Source: CAD feature listing. Evaluate the final solid. Frame: model axes, mm. A direction names the side the tool comes from. Coordinates: 2 decimals unless noted, no trailing zeros. Write each loop counter-clockwise with the first axis right and the second up, starting at its lowest first coordinate (ties: lowest second). Pieces come first, ordered by that corner, then holes. Notation, with made-up numbers: M 78.25,-17 L 106.25,-17 A16 cw 106.25,4 Z; hole C 6.5,-5 d10. An arc over 180 degrees is marked long. Answer as CSV lines item,"result". Start each with the question number.
1. Section B-B on x = 23.5. Return the cut outline in (y, z), plus the area to 3 significant figures.
2. Contact query for flat-ended pins moving along their axis: pin 1 Ø1.2 at (x, y) = (49.5, 7) entering from +Z; pin 2 Ø1.6 at (x, y) = (0.5, 7) entering from -Z; pin 3 Ø1.2 at (x, y) = (49.5, 7) entering from -Z; pin 4 Ø2 at (x, y) = (62.5, 6.5) entering from -Z. Output: stop coordinate, or through.
3. Line query: probe 1 along Z at (x, y) = (39, 0.5); probe 2 along Z at (x, y) = (41.5, 1.75); probe 3 along X at (y, z) = (6.25, -5). Output: solid intervals per line, ascending. Write a range as [from, to].
4. Reachability of faces 1 (the face through (0.76, 2.9, 5.86)), 2 (the face through (42.797, 1.014, 29.359)), 3 (the face through (5, 5, -44.75)), 4 (the face through (7.86, 2.9, -1.01)), 5 (the face through (55.6, 2.86, -46.4)) from +Z, -Z, +X, -X, +Y, -Y: full face, straight path, thin tool, end or side. Return the list, or none.
5. Section A-A on z = 20.5. Return the cut outline in (x, y), plus the area to 3 significant figures.
6. Mould query, pull axis X, two halves, no side actions, for faces 6 (the face through (5, 5, 34.5)), 7 (the face through (3, 8, -45)), 8 (the face through (62.93, 4.06, -0.6)). Classes: pulls with the +X half, pulls with the -X half, needs draft (parallel to the pull), parting line crosses it, or undercut.
7. Section D-D on z = -24.5. Return the cut outline in (x, y).
8. Section C-C on y = 6.5. Count the separate pieces of the cut face and the enclosed holes in it, plus the area to 3 significant figures.
```python
from build123d import *

# Parameters (mm, degrees)
SKETCH1_W            = 63.5
SKETCH1_H            = 48
BOSS_EXTRUDE6_DEPTH  = 21
SKETCH5_W            = 50
SKETCH5_H            = 38.5
BOSS_EXTRUDE7_DEPTH  = 11.5
SKETCH6_W            = 59.5
SKETCH6_H            = 44
CUT_EXTRUDE1_DEPTH   = 19
SKETCH7_W            = 46
SKETCH7_H            = 34.5
CUT_EXTRUDE2_DEPTH   = 9.5
SKETCH8_W            = 50
SKETCH8_H            = 11.5
CUT_EXTRUDE4_DEPTH   = 2
CUT_EXTRUDE6_DEPTH   = 2
CUT_EXTRUDE7_DEPTH   = 2
CUT_EXTRUDE10_DEPTH  = 72
CUT_EXTRUDE11_DEPTH  = 38
SKETCH16_W           = 67
SKETCH16_H           = 6.5
CUT_EXTRUDE13_DEPTH  = 79
CUT_EXTRUDE14_DEPTH  = 79
CUT_EXTRUDE15_DEPTH  = 79
FILLET1_R            = 2
FILLET2_R            = 2
FILLET3_R            = 2
FILLET4_R            = 2
FILLET5_R            = 2
SKETCH19_W           = 36.5
SKETCH19_H           = 2
CUT_EXTRUDE17_DEPTH  = 79
FILLET6_R            = 5
FILLET7_R            = 5
SKETCH20_W           = 4
SKETCH20_H           = 2
BOSS_EXTRUDE16_DEPTH = 18
SKETCH30_W           = 4
SKETCH30_H           = 1
BOSS_EXTRUDE17_DEPTH = 2
SKETCH33_W           = 4
SKETCH33_H           = 1.5
BOSS_EXTRUDE18_DEPTH = 4
SKETCH34_W           = 4
SKETCH34_H           = 1
BOSS_EXTRUDE19_DEPTH = 2
SKETCH36_W           = 4
SKETCH36_H           = 1
CUT_EXTRUDE21_DEPTH  = 2
CUT_EXTRUDE22_DEPTH  = 7
CUT_EXTRUDE25_DEPTH  = 7
SKETCH39_W           = 9.212342007
SKETCH39_H           = 18
CUT_EXTRUDE26_DEPTH  = 10
SKETCH40_W           = 63.5
SKETCH40_H           = 6.5
CUT_EXTRUDE27_DEPTH  = 117
SKETCH44_W           = 34.5
SKETCH44_H           = 6
CUT_EXTRUDE30_DEPTH  = 0.5
SKETCH45_W           = 34.5
SKETCH45_H           = 6
CUT_EXTRUDE31_DEPTH  = 0.5
SKETCH46_W           = 44
SKETCH46_H           = 6
BOSS_EXTRUDE20_DEPTH = 1.25
SKETCH47_W           = 58.25
SKETCH47_H           = 6
BOSS_EXTRUDE21_DEPTH = 1.25
CUT_EXTRUDE32_START  = -1.25
CUT_EXTRUDE32_DEPTH  = 1.25
CUT_EXTRUDE33_DEPTH  = 1.25


with BuildPart() as part:
    # Sketch1 → Boss-Extrude6 (new body)
    with BuildSketch(Plane(origin=(0, 0, 0), x_dir=(1, 0, 0), z_dir=(0, 1, 0))):
        with Locations((31.75, 24)):
            Rectangle(SKETCH1_W, SKETCH1_H)
    extrude(amount=BOSS_EXTRUDE6_DEPTH)

    # Sketch5 → Boss-Extrude7 (add)
    with BuildSketch(Plane(origin=(0, 0, 0), x_dir=(-1, 0, 0), z_dir=(0, -1, 0))):
        with Locations((-25, -19.25)):
            Rectangle(SKETCH5_W, SKETCH5_H)
    extrude(amount=-BOSS_EXTRUDE7_DEPTH)

    # Sketch6 → Cut-Extrude1 (cut)
    with BuildSketch(Plane(origin=(0, 21, 0), x_dir=(1, 0, 0), z_dir=(0, 1, 0))):
        with Locations((31.75, 24)):
            Rectangle(SKETCH6_W, SKETCH6_H)
    extrude(amount=-CUT_EXTRUDE1_DEPTH, mode=Mode.SUBTRACT)

    # Sketch7 → Cut-Extrude2 (cut)
    with BuildSketch(Plane(origin=(0, 11.5, 0), x_dir=(1, 0, 0), z_dir=(0, 1, 0))):
        with Locations((25, -17.25)):
            Rectangle(SKETCH7_W, SKETCH7_H)
    extrude(amount=-CUT_EXTRUDE2_DEPTH, mode=Mode.SUBTRACT)

    # Sketch8 → Cut-Extrude4 (cut)
    with BuildSketch(Plane.XY.offset(38.5)):
        with Locations((25, 5.75)):
            Rectangle(SKETCH8_W, SKETCH8_H)
    extrude(amount=-CUT_EXTRUDE4_DEPTH, mode=Mode.SUBTRACT)

    # Sketch10 → Cut-Extrude6 (cut)
    with BuildSketch(Plane(origin=(0, 2, 0), x_dir=(1, 0, 0), z_dir=(0, 1, 0))):
        with BuildLine():
            Line((12, 7), (51.5, 7))
            ThreePointArc((51.5, 7), (55.035533906, 8.464466094), (56.5, 12))
            Line((56.5, 12), (56.5, 36))
            ThreePointArc((56.5, 36), (55.035533906, 39.535533906), (51.5, 41))
            Line((51.5, 41), (12, 41))
            ThreePointArc((12, 41), (8.464466094, 39.535533906), (7, 36))
            Line((7, 36), (7, 12))
            ThreePointArc((7, 12), (8.464466094, 8.464466094), (12, 7))
        make_face()
    extrude(amount=-CUT_EXTRUDE6_DEPTH, mode=Mode.SUBTRACT)

    # Sketch11 → Cut-Extrude7 (cut)
    with BuildSketch(Plane(origin=(0, 2, 0), x_dir=(1, 0, 0), z_dir=(0, 1, 0))):
        with BuildLine():
            Line((10, -30.5), (40, -30.5))
            ThreePointArc((40, -30.5), (42.828427125, -29.328427125), (44, -26.5))
            Line((44, -26.5), (44, -8))
            ThreePointArc((44, -8), (42.828427125, -5.171572875), (40, -4))
            Line((40, -4), (10, -4))
            ThreePointArc((10, -4), (7.171572875, -5.171572875), (6, -8))
            Line((6, -8), (6, -26.5))
            ThreePointArc((6, -26.5), (7.171572875, -29.328427125), (10, -30.5))
        make_face()
    extrude(amount=-CUT_EXTRUDE7_DEPTH, mode=Mode.SUBTRACT)

    # Sketch13 → Cut-Extrude10 (cut)
    with BuildSketch(Plane(origin=(63.5, 0, 0), x_dir=(0, 0, -1), z_dir=(1, 0, 0))):
        with BuildLine():
            Line((7, 21), (41, 21))
            Line((41, 21), (41, 5))
            ThreePointArc((41, 5), (40.121320344, 2.878679656), (38, 2))
            Line((38, 2), (10, 2))
            ThreePointArc((10, 2), (7.878679656, 2.878679656), (7, 5))
            Line((7, 5), (7, 21))
        make_face()
    extrude(amount=-CUT_EXTRUDE10_DEPTH, mode=Mode.SUBTRACT)

    # Sketch14 → Cut-Extrude11 (cut)
    with BuildSketch(Plane(origin=(0, 0, -48), x_dir=(-1, 0, 0), z_dir=(0, 0, -1))):
        with BuildLine():
            Line((-56.5, 21), (-7, 21))
            Line((-7, 21), (-7, 5))
            ThreePointArc((-7, 5), (-7.878679656, 2.878679656), (-10, 2))
            Line((-10, 2), (-53.5, 2))
            ThreePointArc((-53.5, 2), (-55.621320344, 2.878679656), (-56.5, 5))
            Line((-56.5, 5), (-56.5, 21))
        make_face()
    extrude(amount=-CUT_EXTRUDE11_DEPTH, mode=Mode.SUBTRACT)

    # Sketch16 → Cut-Extrude13 (cut)
    with BuildSketch(Plane(origin=(63.5, 0, 0), x_dir=(0, 0, -1), z_dir=(1, 0, 0))):
        with Locations((14.5, 17.75)):
            Rectangle(SKETCH16_W, SKETCH16_H)
    extrude(amount=-CUT_EXTRUDE13_DEPTH, mode=Mode.SUBTRACT)

    # Sketch17 → Cut-Extrude14 (cut)
    with BuildSketch(Plane(origin=(0, 0, -2), x_dir=(-1, 0, 0), z_dir=(0, 0, -1))):
        with BuildLine():
            Line((-43, 14.5), (-7, 14.5))
            Line((-7, 14.5), (-7, 5))
            ThreePointArc((-7, 5), (-7.878679656, 2.878679656), (-10, 2))
            Line((-10, 2), (-40, 2))
            ThreePointArc((-40, 2), (-42.121320344, 2.878679656), (-43, 5))
            Line((-43, 5), (-43, 14.5))
        make_face()
    extrude(amount=-CUT_EXTRUDE14_DEPTH, mode=Mode.SUBTRACT)

    # Sketch18 → Cut-Extrude15 (cut)
    with BuildSketch(Plane(origin=(50, 0, 0), x_dir=(0, 0, -1), z_dir=(1, 0, 0))):
        with BuildLine():
            Line((-29.5, 11.5), (-5, 11.5))
            Line((-5, 11.5), (-5, 5))
            ThreePointArc((-5, 5), (-5.878679656, 2.878679656), (-8, 2))
            Line((-8, 2), (-26.5, 2))
            ThreePointArc((-26.5, 2), (-28.621320344, 2.878679656), (-29.5, 5))
            Line((-29.5, 5), (-29.5, 11.5))
        make_face()
    extrude(amount=-CUT_EXTRUDE15_DEPTH, mode=Mode.SUBTRACT)

    # Fillet1
    fillet1_edges = [part.edges().sort_by_distance(p)[0] for p in [
        (50, 5.75, 36.5),
    ]]
    fillet(fillet1_edges, radius=FILLET1_R)

    # Fillet2
    fillet2_edges = [part.edges().sort_by_distance(p)[0] for p in [
        (0, 5.75, 36.5),
    ]]
    fillet(fillet2_edges, radius=FILLET2_R)

    # Fillet3
    fillet3_edges = [part.edges().sort_by_distance(p)[0] for p in [
        (0, 7.25, -48),
    ]]
    fillet(fillet3_edges, radius=FILLET3_R)

    # Fillet4
    fillet4_edges = [part.edges().sort_by_distance(p)[0] for p in [
        (63.5, 7.25, -48),
    ]]
    fillet(fillet4_edges, radius=FILLET4_R)

    # Fillet5
    fillet5_edges = [part.edges().sort_by_distance(p)[0] for p in [
        (63.5, 7.25, 0),
    ]]
    fillet(fillet5_edges, radius=FILLET5_R)

    # Sketch19 → Cut-Extrude17 (cut)
    with BuildSketch(Plane(origin=(50, 0, 0), x_dir=(0, 0, -1), z_dir=(1, 0, 0))):
        with Locations((-18.25, 10.5)):
            Rectangle(SKETCH19_W, SKETCH19_H)
    extrude(amount=-CUT_EXTRUDE17_DEPTH, mode=Mode.SUBTRACT)

    # Fillet6
    fillet6_edges = [part.edges().sort_by_distance(p)[0] for p in [
        (1, 9.5, 0),
    ]]
    fillet(fillet6_edges, radius=FILLET6_R - 0.0001)  # a hair under: the kernel refuses the full size

    # Fillet7
    fillet7_edges = [part.edges().sort_by_distance(p)[0] for p in [
        (49, 9.5, 0),
    ]]
    fillet(fillet7_edges, radius=FILLET7_R - 0.0001)  # a hair under: the kernel refuses the full size

    # Sketch20 → Boss-Extrude16 (add)
    with BuildSketch(Plane(origin=(0, 2, 0), x_dir=(1, 0, 0), z_dir=(0, 1, 0))):
        with Locations((25, 1)):
            Rectangle(SKETCH20_W, SKETCH20_H)
    extrude(amount=BOSS_EXTRUDE16_DEPTH)

    # Sketch30 → Boss-Extrude17 (add)
    with BuildSketch(Plane.XY):
        with Locations((25, 19.5)):
            Rectangle(SKETCH30_W, SKETCH30_H)
    extrude(amount=BOSS_EXTRUDE17_DEPTH)

    # Sketch33 → Boss-Extrude18 (add)
    with BuildSketch(Plane.XY):
        with Locations((25, 12.75)):
            Rectangle(SKETCH33_W, SKETCH33_H)
    extrude(amount=BOSS_EXTRUDE18_DEPTH)

    # Sketch34 → Boss-Extrude19 (add)
    with BuildSketch(Plane(origin=(0, 0, -2), x_dir=(-1, 0, 0), z_dir=(0, 0, -1))):
        with Locations((-25, 19.5)):
            Rectangle(SKETCH34_W, SKETCH34_H)
    extrude(amount=BOSS_EXTRUDE19_DEPTH)

    # Sketch36 → Cut-Extrude21 (cut)
    with BuildSketch(Plane.XY.offset(2)):
        with Locations((25, 19.5)):
            Rectangle(SKETCH36_W, SKETCH36_H)
    extrude(amount=-CUT_EXTRUDE21_DEPTH, mode=Mode.SUBTRACT)

    # Sketch37 → Cut-Extrude22 (cut)
    with BuildSketch(Plane(origin=(27, 0, 0), x_dir=(0, 0, -1), z_dir=(1, 0, 0))):
        Polygon((0, 20), (4, 19.257089557), (4, 20), align=None)
    extrude(amount=-CUT_EXTRUDE22_DEPTH, mode=Mode.SUBTRACT)

    # Sketch38 → Cut-Extrude25 (cut)
    with BuildSketch(Plane(origin=(27, 0, 0), x_dir=(0, 0, -1), z_dir=(1, 0, 0))):
        Polygon((0, 13.5), (-4, 10.225610037), (-4, 13.5), align=None)
    extrude(amount=-CUT_EXTRUDE25_DEPTH, mode=Mode.SUBTRACT)

    # Sketch39 → Cut-Extrude26 (cut)
    with BuildSketch(Plane(origin=(27, 0, 0), x_dir=(0, 0, -1), z_dir=(1, 0, 0))):
        with Locations((2.773768612, 11)):
            Rectangle(SKETCH39_W, SKETCH39_H)
    extrude(amount=-CUT_EXTRUDE26_DEPTH, mode=Mode.SUBTRACT)

    # Sketch40 → Cut-Extrude27 (cut)
    with BuildSketch(Plane(origin=(0, 0, -48), x_dir=(-1, 0, 0), z_dir=(0, 0, -1))):
        with Locations((-31.75, 11.25)):
            Rectangle(SKETCH40_W, SKETCH40_H)
    extrude(amount=-CUT_EXTRUDE27_DEPTH, mode=Mode.SUBTRACT)

    # Sketch44 → Cut-Extrude30 (cut)
    with BuildSketch(Plane(origin=(2, 0, 0), x_dir=(0, 0, -1), z_dir=(1, 0, 0))):
        with Locations((-17.25, 5)):
            Rectangle(SKETCH44_W, SKETCH44_H)
    extrude(amount=-CUT_EXTRUDE30_DEPTH, mode=Mode.SUBTRACT)

    # Sketch45 → Cut-Extrude31 (cut)
    with BuildSketch(Plane.ZY.offset(-48)):
        with Locations((17.25, 5)):
            Rectangle(SKETCH45_W, SKETCH45_H)
    extrude(amount=-CUT_EXTRUDE31_DEPTH, mode=Mode.SUBTRACT)

    # Sketch46 → Boss-Extrude20 (add)
    with BuildSketch(Plane(origin=(2, 0, 0), x_dir=(0, 0, -1), z_dir=(1, 0, 0))):
        with Locations((24, 5)):
            Rectangle(SKETCH46_W, SKETCH46_H)
    extrude(amount=BOSS_EXTRUDE20_DEPTH)

    # Sketch47 → Boss-Extrude21 (add)
    with BuildSketch(Plane.XY.offset(-46)):
        with Locations((32.375, 5)):
            Rectangle(SKETCH47_W, SKETCH47_H)
    extrude(amount=BOSS_EXTRUDE21_DEPTH)

    # Sketch48 → Cut-Extrude32 (cut)
    with BuildSketch(Plane.ZY.offset(-2).offset(CUT_EXTRUDE32_START)):
        with BuildLine():
            Line((-7, 8), (-41, 8))
            Line((-41, 8), (-41, 5))
            ThreePointArc((-41, 5), (-40.121320344, 2.878679656), (-38, 2))
            Line((-38, 2), (-10, 2))
            ThreePointArc((-10, 2), (-7.878679656, 2.878679656), (-7, 5))
            Line((-7, 5), (-7, 8))
        make_face()
    extrude(amount=CUT_EXTRUDE32_DEPTH, mode=Mode.SUBTRACT)

    # Sketch49 → Cut-Extrude33 (cut)
    with BuildSketch(Plane(origin=(0, 0, -46), x_dir=(-1, 0, 0), z_dir=(0, 0, -1))):
        with BuildLine():
            Line((-7, 8), (-56.5, 8))
            Line((-56.5, 8), (-56.5, 5))
            ThreePointArc((-56.5, 5), (-55.621320344, 2.878679656), (-53.5, 2))
            Line((-53.5, 2), (-10, 2))
            ThreePointArc((-10, 2), (-7.878679656, 2.878679656), (-7, 5))
            Line((-7, 5), (-7, 8))
        make_face()
    extrude(amount=-CUT_EXTRUDE33_DEPTH, mode=Mode.SUBTRACT)


solid = part.part
```
Values:
1,outline,"M 0,-48 L 2,-48 L 2,-41 L 0,-41 Z; M 0,-7 L 2,-7 L 2,4 L 0,4 Z; M 0,30.5 L 2,30.5 L 2,36.5 L 0,36.5 Z"
1,area,"48.0 mm²"
2,pin 1,"z = 36.29"
2,pin 2,"z = -47.87"
2,pin 3,"z = -2"
2,pin 4,"z = -48"
3,probe 1,"[-48, -41], [-7, 4], [30.5, 36.5]"
3,probe 2,"[-48, -41], [-7, 4.29], [30.21, 36.5]"
3,probe 3,"[0, 3.25], [61.5, 63.5]"
4,face 1,"+X, -X, +Y"
4,face 2,"+Y, -Y"
4,face 3,"+Y"
4,face 4,"+Z, -Z, +Y"
4,face 5,"-Z, +Y"
5,outline,"M 0,0 L 6,0 L 6,2 L 0,2 Z; M 44,0 L 50,0 L 50,2 L 44,2 Z"
5,area,"24.0 mm²"
6,face 6,"undercut"
6,face 7,"needs draft"
6,face 8,"pulls with the +X half"
7,outline,"M 0,0 L 7,0 L 7,2 L 0,2 Z; M 56.5,0 L 63.5,0 L 63.5,2 L 56.5,2 Z"
8,separate pieces,"6"
8,enclosed holes,"0"
8,area,"200 mm²"
